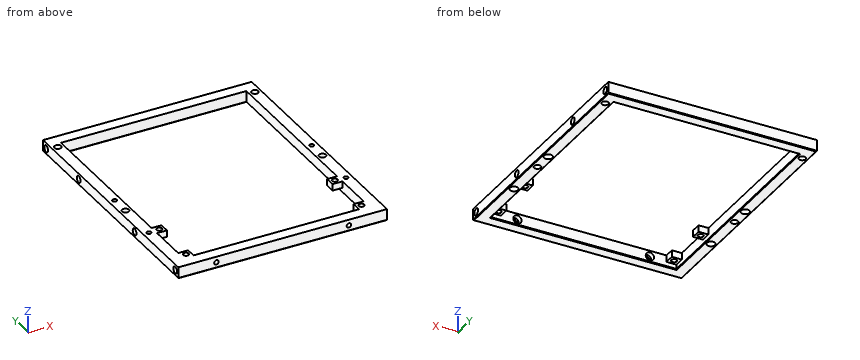
from build123d import *

# Parameters (mm, degrees)
SKETCH1_W           = 126
SKETCH1_H           = 150
SKETCH1_W_2         = 112
SKETCH1_H_2         = 136
BOSS_EXTRUDE1_DEPTH = 7
SKETCH2_R           = 2.05
CUT_EXTRUDE1_DEPTH  = 6
SKETCH3_R           = 1.35
CUT_EXTRUDE2_DEPTH  = 8
SKETCH4_R           = 2.5
CUT_EXTRUDE3_DEPTH  = 3
SKETCH5_R           = 1.35
CUT_EXTRUDE4_DEPTH  = 8
SKETCH6_R           = 2.5
CUT_EXTRUDE5_DEPTH  = 3
SKETCH7_R           = 2.05
CUT_EXTRUDE6_DEPTH  = 8
CUT_EXTRUDE7_DEPTH  = 0.2
SKETCH9_W           = 2.7
SKETCH9_H           = 2.7
CUT_EXTRUDE8_DEPTH  = 0.2
SKETCH10_W          = 6
SKETCH10_H          = 6
BOSS_EXTRUDE2_DEPTH = 4
SKETCH11_R          = 1.65
CUT_EXTRUDE9_DEPTH  = 5
CHAMFER1_SIZE       = 0.4
CHAMFER2_SIZE       = 0.4


with BuildPart() as part:
    # Sketch1 → Boss-Extrude1 (new body)
    with BuildSketch(Plane.XY):
        Rectangle(SKETCH1_W, SKETCH1_H)
        Rectangle(SKETCH1_W_2, SKETCH1_H_2, mode=Mode.SUBTRACT)
    extrude(amount=BOSS_EXTRUDE1_DEPTH)

    # Sketch2 → Cut-Extrude1 (cut)
    with BuildSketch(Plane.ZY.offset(63)):
        with Locations((3.5, -71.5)):
            Circle(SKETCH2_R)
        with Locations((3.5, 71.5)):
            Circle(SKETCH2_R)
        with Locations((3.5, 35.5)):
            Circle(SKETCH2_R)
        with Locations((3.5, -26.5)):
            Circle(SKETCH2_R)
    cut_extrude1 = extrude(amount=-CUT_EXTRUDE1_DEPTH, mode=Mode.SUBTRACT)

    # Mirror1: Cut-Extrude1 across plane
    add(cut_extrude1.mirror(Plane(origin=(0, 0, 0), x_dir=(0, 0, 1), z_dir=(1, 0, 0))), mode=Mode.SUBTRACT)

    # Sketch3 → Cut-Extrude2 (cut, through all)
    with BuildSketch(Plane(origin=(0, -68, 0), x_dir=(1, 0, 0), z_dir=(0, 1, 0))):
        with Locations((40, -3.5)):
            Circle(SKETCH3_R)
        with Locations((-40, -3.5)):
            Circle(SKETCH3_R)
    extrude(amount=-CUT_EXTRUDE2_DEPTH, mode=Mode.SUBTRACT)

    # Sketch4 → Cut-Extrude3 (cut)
    with BuildSketch(Plane(origin=(0, -68, 0), x_dir=(1, 0, 0), z_dir=(0, 1, 0))):
        with Locations((40, -3.5)):
            Circle(SKETCH4_R)
        with Locations((-40, -3.5)):
            Circle(SKETCH4_R)
    extrude(amount=-CUT_EXTRUDE3_DEPTH, mode=Mode.SUBTRACT)

    # Sketch5 → Cut-Extrude4 (cut, through all)
    with BuildSketch(Plane(origin=(0, 0, 0), x_dir=(-1, 0, 0), z_dir=(0, 0, -1))):
        with Locations((-59.5, 2)):
            Circle(SKETCH5_R)
        with Locations((59.5, 2)):
            Circle(SKETCH5_R)
        with Locations((-59.5, -36)):
            Circle(SKETCH5_R)
        with Locations((59.5, -36)):
            Circle(SKETCH5_R)
    extrude(amount=-CUT_EXTRUDE4_DEPTH, mode=Mode.SUBTRACT)

    # Sketch6 → Cut-Extrude5 (cut)
    with BuildSketch(Plane(origin=(0, 0, 0), x_dir=(-1, 0, 0), z_dir=(0, 0, -1))):
        with Locations((-59.5, 2)):
            Circle(SKETCH6_R)
        with Locations((59.5, 2)):
            Circle(SKETCH6_R)
        with Locations((-59.5, -36)):
            Circle(SKETCH6_R)
        with Locations((59.5, -36)):
            Circle(SKETCH6_R)
    extrude(amount=-CUT_EXTRUDE5_DEPTH, mode=Mode.SUBTRACT)

    # Sketch7 → Cut-Extrude6 (cut, through all)
    with BuildSketch(Plane(origin=(0, 0, 0), x_dir=(-1, 0, 0), z_dir=(0, 0, -1))):
        with Locations((-59.5, 65)):
            Circle(SKETCH7_R)
        with Locations((-59.5, -10)):
            Circle(SKETCH7_R)
    cut_extrude6 = extrude(amount=-CUT_EXTRUDE6_DEPTH, mode=Mode.SUBTRACT)

    # Mirror2: Cut-Extrude6 across plane
    add(cut_extrude6.mirror(Plane(origin=(0, 0, 0), x_dir=(0, 0, 1), z_dir=(1, 0, 0))), mode=Mode.SUBTRACT)

    # Sketch8 → Cut-Extrude7 (cut)
    with BuildSketch(Plane(origin=(0, 0, 3), x_dir=(-1, 0, 0), z_dir=(0, 0, -1))):
        with BuildLine():
            Line((-60.85, -0.104162541), (-60.85, 4.104162541))
            ThreePointArc((-60.85, 4.104162541), (-59.5, 4.5), (-58.15, 4.104162541))
            Line((-58.15, 4.104162541), (-58.15, -0.104162541))
            ThreePointArc((-58.15, -0.104162541), (-59.5, -0.5), (-60.85, -0.104162541))
        make_face()
        with BuildLine():
            Line((-60.85, -38.104162541), (-60.85, -33.895837459))
            ThreePointArc((-60.85, -33.895837459), (-59.5, -33.5), (-58.15, -33.895837459))
            Line((-58.15, -33.895837459), (-58.15, -38.104162541))
            ThreePointArc((-58.15, -38.104162541), (-59.5, -38.5), (-60.85, -38.104162541))
        make_face()
    cut_extrude7 = extrude(amount=-CUT_EXTRUDE7_DEPTH, mode=Mode.SUBTRACT)

    # Sketch9 → Cut-Extrude8 (cut)
    with BuildSketch(Plane(origin=(0, 0, 3.2), x_dir=(-1, 0, 0), z_dir=(0, 0, -1))):
        with Locations((-59.5, 2)):
            Rectangle(SKETCH9_W, SKETCH9_H)
        with Locations((-59.5, -36)):
            Rectangle(SKETCH9_W, SKETCH9_H)
    cut_extrude8 = extrude(amount=-CUT_EXTRUDE8_DEPTH, mode=Mode.SUBTRACT)

    # Mirror3: Cut-Extrude7, Cut-Extrude8 across plane
    add(cut_extrude7.mirror(Plane(origin=(0, 0, 0), x_dir=(0, 0, 1), z_dir=(1, 0, 0))), mode=Mode.SUBTRACT)
    add(cut_extrude8.mirror(Plane(origin=(0, 0, 0), x_dir=(0, 0, 1), z_dir=(1, 0, 0))), mode=Mode.SUBTRACT)

    # Sketch10 → Boss-Extrude2 (add)
    with BuildSketch(Plane.XY.offset(7)):
        with Locations((53, -65)):
            Rectangle(SKETCH10_W, SKETCH10_H)
        with Locations((53, -35.5)):
            Rectangle(SKETCH10_W, SKETCH10_H)
    boss_extrude2 = extrude(amount=-BOSS_EXTRUDE2_DEPTH)

    # Sketch11 → Cut-Extrude9 (cut, through all)
    with BuildSketch(Plane(origin=(0, 0, 3), x_dir=(-1, 0, 0), z_dir=(0, 0, -1))):
        with Locations((-53, -35.5)):
            Circle(SKETCH11_R)
        with Locations((-53, -65)):
            Circle(SKETCH11_R)
    cut_extrude9 = extrude(amount=-CUT_EXTRUDE9_DEPTH, mode=Mode.SUBTRACT)

    # Mirror4: Boss-Extrude2, Cut-Extrude9 across plane
    add(boss_extrude2.mirror(Plane(origin=(0, 0, 0), x_dir=(0, 0, 1), z_dir=(1, 0, 0))))
    add(cut_extrude9.mirror(Plane(origin=(0, 0, 0), x_dir=(0, 0, 1), z_dir=(1, 0, 0))), mode=Mode.SUBTRACT)

    # Chamfer1
    chamfer1_edges = [part.edges().sort_by_distance(p)[0] for p in [
        (56, 0, 0),
        (0, 68, 0),
        (-56, 0, 0),
        (0, -68, 0),
    ]]
    chamfer(chamfer1_edges, length=CHAMFER1_SIZE)

    # Chamfer2
    chamfer2_edges = [part.edges().sort_by_distance(p)[0] for p in [
        (0, -75, 0),
        (-63, 0, 0),
        (0, 75, 0),
        (63, 0, 0),
    ]]
    chamfer(chamfer2_edges, length=CHAMFER2_SIZE)


solid = part.part
Build history of the part. All positions in model axes, mm. Give positions to 0.01 mm unless a question says otherwise; leave off trailing zeros. Order: outer loops, then holes, each group sorted by start corner. A loop starts at its lowest first (then second) coordinate and runs counter-clockwise, first axis right, second up. Notation, with made-up numbers: M 2,65 L 44,65 A35 cw 44,101 Z; hole C 47.5,13 d3. An arc over 180 degrees is marked long. Put each result on its own line as item: value.
Item 1: Slice it at D-D, the plane y = -65. Write the cut outline in (x, z), plus the area to 3 significant figures.
From the geometry:
outline: M -63,0.4 L -62.6,0 L -56.4,0 L -56,0.4 L -56,3 L -54.65,3 L -54.65,7 L -63,7 Z; M -51.35,3 L -50,3 L -50,7 L -51.35,7 Z; M 50,3 L 51.35,3 L 51.35,7 L 50,7 Z; M 54.65,3 L 56,3 L 56,0.4 L 56.4,0 L 62.6,0 L 63,0.4 L 63,7 L 54.65,7 Z
area: 119 mm2
Item 2: Flat gauge pins, fed straight in: pin 1 Ø3 at (x, y) = (54, -36.5) entering from -Z; pin 2 Ø1.2 at (y, z) = (-27, 4) entering from -X; pin 3 Ø0.9 at (x, y) = (-59.5, 0) entering from -Z; pin 4 Ø2 at (x, y) = (-59.5, -36) entering from +Z. Where does each tip first touch, or does it go through?
From the geometry:
pin 1: stops at z = 3
pin 2: stops at x = -57
pin 3: stops at z = 3.2
pin 4: passes through
Item 3: Slice it at C-C, the plane y = -10. Write the cut outline in (x, z).
From the geometry:
outline: M -63,0.4 L -62.6,0 L -61.55,0 L -61.55,7 L -63,7 Z; M -57.45,0 L -56.4,0 L -56,0.4 L -56,7 L -57.45,7 Z; M 56,0.4 L 56.4,0 L 57.45,0 L 57.45,7 L 56,7 Z; M 61.55,0 L 62.6,0 L 63,0.4 L 63,7 L 61.55,7 Z
Item 4: Slice it at A-A, the plane y = 35.5. Write the cut outline in (x, z).
From the geometry:
outline: M -63,0.4 L -62.6,0 L -56.4,0 L -56,0.4 L -56,7 L -63,7 L -63,5.55 L -57,5.55 L -57,1.45 L -63,1.45 Z; M 56,0.4 L 56.4,0 L 62.6,0 L 63,0.4 L 63,1.45 L 57,1.45 L 57,5.55 L 63,5.55 L 63,7 L 56,7 Z
Item 5: Slice it at B-B, the plane x = -28.5. Write the cut outline in (y, z).
From the geometry:
outline: M -75,0.4 L -74.6,0 L -68.4,0 L -68,0.4 L -68,7 L -75,7 Z; M 68,0.4 L 68.4,0 L 74.6,0 L 75,0.4 L 75,7 L 68,7 Z
Item 6: Probe line 1 (Y direction, x = -50.5, z = 6); line 2 (X direction, y = -65, z = 4.7); line 3 (Y direction, x = 16.5, z = 1.25). List the from-to ranges inside material, lowest first. Write a range as [from, to].
From the geometry:
line 1: y = [-75, -62], [-38.5, -32.5], [68, 75]
line 2: x = [-63, -54.65], [-51.35, -50], [50, 51.35], [54.65, 63]
line 3: y = [-75, -68], [68, 75]
